Verification items for the finished model (mm, model axes). Round coordinates to 2 decimals unless told otherwise and drop trailing zeros. Order: outer loops, then holes, each group sorted by start corner. A loop starts at its lowest first (then second) coordinate and runs counter-clockwise, first axis right, second up. Notation, with made-up numbers: (37.25, -29) -> (48.25, -29) arc R25 cw to (48.25, -2) -> close; hole circle Ø6 at (19, 17.5). An arc over 180 degrees is marked (long way). Return JSON: item names as keys, results as strings. Group by question number.
Item 1: Scan lines: probe 1 along Y at (x, z) = (3.5, 105) (3 decimals); probe 2 along Y at (x, z) = (3.25, 76.5); probe 3 along X at (y, z) = (50.5, 96.5). Record each from-to range of solid material in increasing order. Write a range as from..to.
Item 2: Sectioned sample at C-C on y = 25. Record the cut outline in (x, z), plus the area to 3 significant figures.
Item 3: Depth check by flat-ended pin: pin 1 Ø1 at (x, z) = (3, 77) entering from -Y; pin 2 Ø5 at (x, y) = (-3, 28) entering from +Z; pin 3 Ø5 at (x, y) = (-3.5, 0.5) entering from +Z; pin 4 Ø2 at (x, y) = (1.5, 2.5) entering from -Z. Enter the tip coordinate at first touch or a pass-through.
Item 4: Sectioned sample at B-B on x = 2. Record the cut outline in (y, z), plus the area to 3 significant figures.
Item 5: Sectioned sample at A-A on z = 19. Record the cut outline in (x, y).
Autodesk Inventor part; units mm, degrees
ref_plane "YZ Plane" through (0, 0, 0) normal (1, 0, 0) x (0, 1, 0)
ref_plane "XZ Plane" through (0, 0, 0) normal (0, 1, 0) x (-1, 0, 0)
ref_plane "XY Plane" through (0, 0, 0) normal (0, 0, 1) x (1, 0, 0)
sketch "Sketch3" plane through (0, 0, 0) normal (0, 0, 1) x (1, 0, 0)
  arc A0 (4, 0) -> (-4, 0) centre (0, 0) ccw
  line L0 (5, -0.9717) -> (5, -6.9717)
  line L1 (-5, -6.9717) -> (-5, 0)
  line L2 (-4, 0) -> (-4, -6.9717)
  line L3 (4, 0) -> (4, -6.9717)
  line L4 (5, -6.9717) -> (4, -6.9717)
  line L5 (-4, -6.9717) -> (-5, -6.9717)
  line L6 (-5, 0) -> (-5, 6)
  line L7 (-5, 6) -> (5, 6)
  line L8 (5, 6) -> (5, -0.9717)
  dimension "d9" = 8
  dimension "d11" = 6
  dimension "d29" = 10
  dimension "d30" = 6
sketch "Sketch17" plane through (0, 0, 0) normal (1, 0, 0) x (0, 1, 0)
  line L0 (0, 0) -> (0, 100)
  line L1 (50, 100) -> (50, 0)
  arc A0 (50, 100) -> (0, 100) centre (25, 100) ccw
  dimension "d49" = 100
  dimension "d50" = 50
  dimension "d51" = 50
sweep "Sweep1" add profiles "Sketch3" path "Sketch17"
fillet "Fillet6" radius 5 3 edges at (5, 6, 50) (5, 25, 119) (5, 44, 50)
properties part number "Filament Guide"
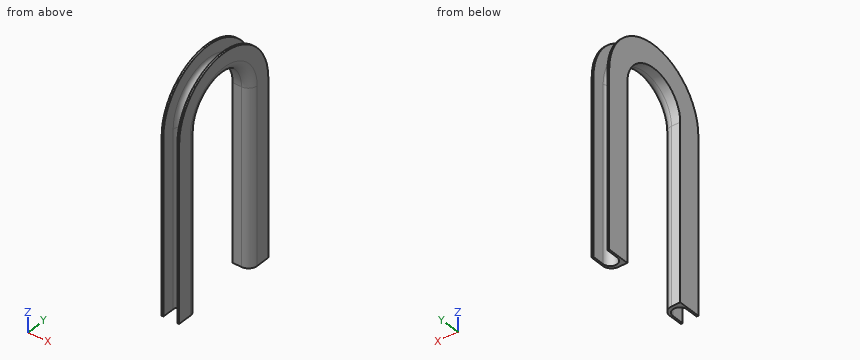
Recorded:
{
 "1": {"probe 1": "2.485..5.192, 44.808..47.515", "probe 2": "2.33..4.8, 45.2..47.67", "probe 3": "-5..-4, 4..5"},
 "2": {"outline": "(-5, 119) -> (0, 119) arc R5 ccw to (5, 124) -> (5, 131.97) -> (4, 131.97) -> (4, 125) arc R4 cw to (-4, 125) -> (-4, 131.97) -> (-5, 131.97) -> close", "area": "43.4 mm²"},
 "3": {"pin 1": "y = 1.94", "pin 2": "z = 131.96", "pin 3": "z = 123.15", "pin 4": "through"},
 "4": {"outline": "(3.46, 0) -> (5.58, 0) -> (5.58, 100) arc R19.42 cw to (44.42, 100) -> (44.42, 0) -> (46.54, 0) -> (46.54, 100) arc R21.54 ccw to (3.46, 100) -> close", "area": "560 mm²"},
 "5": {"outline": "(-5, -6.97) -> (-4, -6.97) -> (-4, 0) arc R4 cw to (4, 0) -> (4, -6.97) -> (5, -6.97) -> (5, 1) arc R5 ccw to (0, 6) -> (-5, 6) -> close; (-5, 44) -> (0, 44) arc R5 ccw to (5, 49) -> (5, 56.97) -> (4, 56.97) -> (4, 50) arc R4 cw to (-4, 50) -> (-4, 56.97) -> (-5, 56.97) -> close"}
}
